Solid Edge part; units mm, degrees
sketch "Sketch1" plane through (0, 0, 0) normal (0, -1, 0) x (1, 0, 0)
  line L0 (37.6, 0) -> (37.6, 580)
  arc A0 (37.6, 580) -> (-37.6, 580) centre (0, 580) ccw
  line L1 (-37.6, 580) -> (-37.6, 0)
  arc A1 (-37.6, 0) -> (37.6, 0) centre (0, 0) ccw
  line L2 (34.6, 580) -> (34.6, 0)
  arc A2 (-34.6, 580) -> (34.6, 580) centre (0, 580) cw
  line L3 (-34.6, 580) -> (-34.6, 0)
  arc A3 (34.6, 0) -> (-34.6, 0) centre (0, 0) cw
extrude "Protrusion1" add sketch "Sketch1" along normal blind 20
sketch "Sketch2" plane through (0, 0, 0) normal (0, -1, 0) x (1, 0, 0)
  line L0 (33.2, 0.6528) -> (33.2, 1.8528)
  line L1 (33.2, 1.8528) -> (34.6, 2.5057)
  line L2 (34.6, 2.5057) -> (34.6, 0)
  line L3 (34.6, 0) -> (33.2, 0.6528)
extrude "Extrusionsausprägung_2" add sketch "Sketch2" along normal blind 20
pattern "Pattern1" [suppressed]
mirror "Mirror1" [suppressed]
The listing builds one solid part. Answer for the finished solid, in the listing's coordinates (mm). A direction names the side the tool comes from. Coordinates: 2 decimals unless noted, no trailing zeros. Loops run counter-clockwise (first coordinate to the right, second up) from the corner with the lowest first, then second, coordinate; pieces in that order, holes last. Notation, with made-up numbers: (76.5, 83.5) -> (120.5, 83.5) arc R7 ccw to (120.5, 95.5) -> close; hole circle Ø9 at (62.25, 29). An arc over 180 degrees is marked (long way). Answer in a Markdown table with one row per item. Add a question column.
1. The part is cut by section A-A, the plane z = 495. Write down the section's boundary in (x, y), then the cut area to 3 significant figures.
2. The part is cut by section C-C, the plane y = -9.5. Write down the section's boundary in (x, z), then the cut area to 3 significant figures.
3. The part is cut by section B-B, the plane x = 0. Write down the section's boundary in (y, z).
4. Flat-ended cylindrical pins translate along their axes: P1, Ø3, axis at x = 21, y = -3.5, coming from the -Z side; P2, Ø1, axis at x = 8, y = -7.5, coming from the +Z side. Find the tip coordinate at first contact, or state that the pin passes through.
5. Consider line 1 (X direction, y = -6.5, z = 66); line 2 (Z direction, x = -2.5, y = -18); line 3 (Z direction, x = 20, y = -4.25). Determine where each line is inside the solid, lowest interval first. Write a range as [from, to].
6. Determine the mould class of faces 3 (the cylindrical face through (0.83, -9.86, -37.59)), 4 (the flat face through (-37.6, -10, 294)), 5 (the cylindrical face through (-0.76, -9.86, 614.59)) for opening direction X: +X half, -X half, draft (parallel to the pull), parting line (faces both ways), or undercut.
7. For faces 1 (the flat face through (34.6, -10, 295)), 2 (the flat face through (37.6, -10, 286)), determine the directions among +Z, -Z, +X, -X, +Y, -Y from which every point of the face is accessible in a straight line to the end or side of a thin tool.
Answer below:
| question | item | result |
|---|---|---|
| 1 | outline | (-37.6, -20) -> (-34.6, -20) -> (-34.6, 0) -> (-37.6, 0) -> close; (34.6, -20) -> (37.6, -20) -> (37.6, 0) -> (34.6, 0) -> close |
| 1 | area | 120 mm2 |
| 2 | outline | (-37.6, 0) arc R37.6 ccw to (37.6, 0) -> (37.6, 580) arc R37.6 ccw to (-37.6, 580) -> close; hole (-34.6, 0) arc R34.6 ccw to (34.6, 0) -> (33.2, 0.65) -> (33.2, 1.85) -> (34.6, 2.51) -> (34.6, 580) arc R34.6 ccw to (-34.6, 580) -> close |
| 2 | area | 4,160 mm2 |
| 3 | outline | (-20, -37.6) -> (0, -37.6) -> (0, -34.6) -> (-20, -34.6) -> close; (-20, 614.6) -> (0, 614.6) -> (0, 617.6) -> (-20, 617.6) -> close |
| 4 | P1 | z = -32.15 |
| 4 | P2 | z = 616.84 |
| 5 | line 1 | [-37.6, -34.6], [34.6, 37.6] |
| 5 | line 2 | [-37.52, -34.51], [614.51, 617.52] |
| 5 | line 3 | [-31.84, -28.23], [608.23, 611.84] |
| 6 | face 3 | parting line |
| 6 | face 4 | -X half |
| 6 | face 5 | undercut |
| 7 | face 1 | +Y, -Y |
| 7 | face 2 | +Z, -Z, +X, +Y, -Y |
